Source: three-view drawing plus pictorial views. Frame: mm from the lowest corner of the part. Give positions to 0.01 mm unless a question says otherwise; leave off trailing zeros. Order: outer loops, then holes, each group sorted by start corner. A loop starts at its lowest first (then second) coordinate and runs counter-clockwise, first axis right, second up. Notation, with made-up numbers: M 3.25,85 L 28.25,85 A17 ccw 28.25,92 Z; hole C 42.25,42.5 d8. An arc over 180 degrees is marked long. One line per item, written item: value. Start each with the question number.
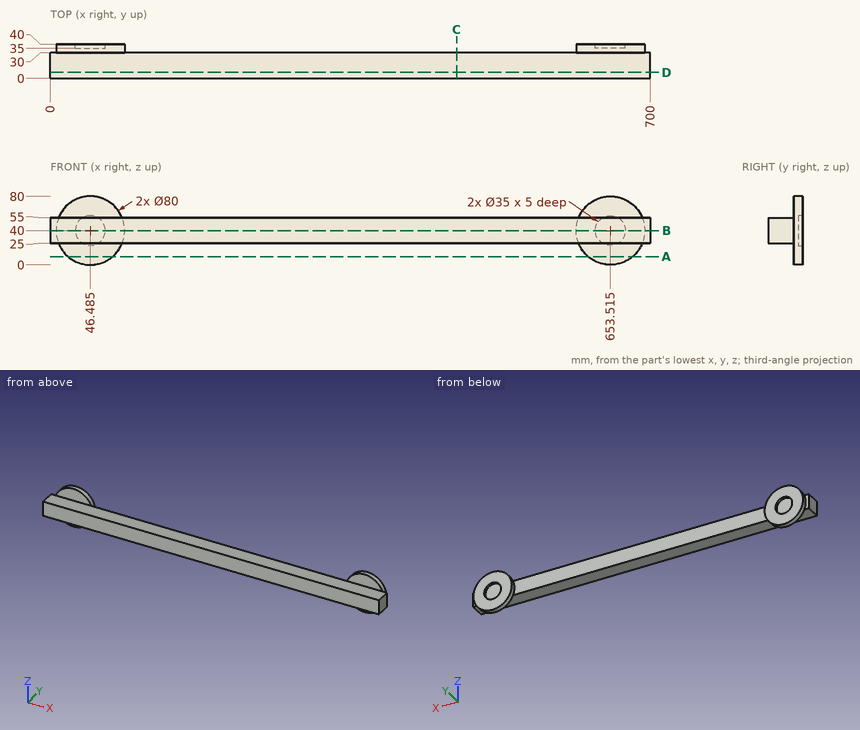
Q1. Section query D-D on y = 7. Return loops of the section in (x, z).
Q2. Ray query, line 1 along X through (y, z) = (38, 40) (1 decimal); line 2 along X through (y, z) = (37.5, 50.5) (1 decimal); line 3 along Z through (x, y) = (189.5, 14). Return the intervals inside material, ascending. Write a range as [from, to].
Q3. Section query A-A on z = 9.5. Return loops of the section in (x, y) (1 decimal), and give its area (4 significant figures).
Q4. Section query C-C on x = 474. Return loops of the section in (y, z).
Q5. Section query B-B on z = 40. Return loops of the section in (x, y) (1 decimal).
Q6. Contact query for flat-ended pins moving along their axis: pin 1 (12 mm diameter, centred on x = 498, z = 23, fed in from +Y); pin 2 (21 mm diameter, centred on x = 653.51, z = 40, fed in from +Y); pin 3 (12 mm diameter, centred on x = 355, y = 11.5, fed in from +Z). Output: stop coordinate, or through.
Results below:
1. outline: M 0,25 L 700,25 L 700,55 L 0,55 Z
2. line 1: [6.5, 29], [64, 86.5], [613.5, 636], [671, 693.5]
2. line 2: [7.9, 32.5], [60.5, 85.1], [614.9, 639.5], [667.5, 692.1]
2. line 3: [25, 55]
3. outline: M 20.6,30 L 72.4,30 L 72.4,40 L 20.6,40 Z; M 627.6,30 L 679.4,30 L 679.4,40 L 627.6,40 Z
3. area: 1,035 mm2
4. outline: M 0,25 L 30,25 L 30,55 L 0,55 Z
5. outline: M 0,0 L 700,0 L 700,30 L 693.5,30 L 693.5,40 L 671,40 L 671,35 L 636,35 L 636,40 L 613.5,40 L 613.5,30 L 86.5,30 L 86.5,40 L 64,40 L 64,35 L 29,35 L 29,40 L 6.5,40 L 6.5,30 L 0,30 Z
6. pin 1: y = 30
6. pin 2: y = 35
6. pin 3: z = 55
